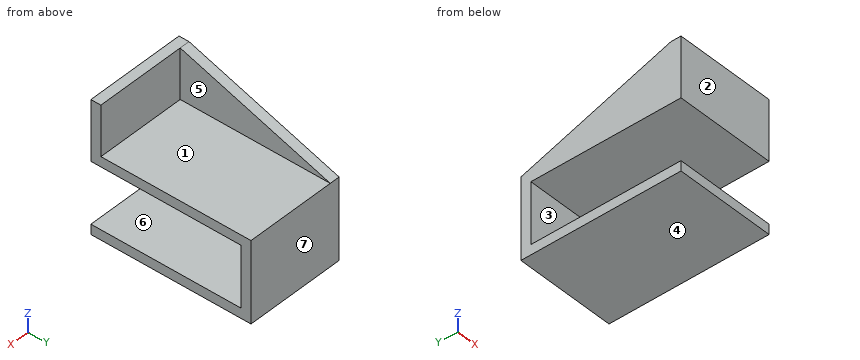
```python
from build123d import *

# Parameters (mm, degrees)
F0_W     = 25
F0_H     = 2.5
F1_DEPTH = 30.5
F2_W     = 50
F2_H     = 80
F3_DEPTH = 5
F4_W     = 50
F4_H     = 5
F5_DEPTH = 25
F7_DEPTH = 5
F8_W     = 50
F8_H     = 5
F9_DEPTH = 80


with BuildPart() as f1:
    # F0 (on Top) → F1 (new body)
    with BuildSketch(Plane.XY):
        with Locations((-12.5, 1.25)):
            Rectangle(F0_W, F0_H)
        with Locations((12.5, 1.25)):
            Rectangle(F0_W, F0_H)
        with Locations((-12.5, -1.25)):
            Rectangle(F0_W, F0_H)
        with Locations((12.5, -1.25)):
            Rectangle(F0_W, F0_H)
    extrude(amount=F1_DEPTH)

    # F2 (on face) → F3 (join)
    with BuildSketch(Plane.XY.offset(30.5)):
        with Locations((0, -37.5)):
            Rectangle(F2_W, F2_H)
    extrude(amount=F3_DEPTH)

    # F4 (on face) → F5 (join)
    with BuildSketch(Plane.XY.offset(35.5)):
        with Locations((0, -75)):
            Rectangle(F4_W, F4_H)
    extrude(amount=F5_DEPTH)

    # F6 (on face) → F7 (join)
    with BuildSketch(Plane(origin=(-25, 0, 0), x_dir=(0, -1, 0), z_dir=(-1, 0, 0))):
        Polygon((77.5, 30.5), (77.5, 60.5), (72.5, 60.5), (-2.5, 35.5), align=None)
    extrude(amount=-F7_DEPTH)

    # F8 (on face) → F9 (join, through all)
    with BuildSketch(Plane(origin=(0, 2.5, 0), x_dir=(-1, 0, 0), z_dir=(0, 1, 0))):
        with Locations((0, -2.5)):
            Rectangle(F8_W, F8_H)
    extrude(amount=-F9_DEPTH)


solid = f1.part
```
Geometry: final body of the model. Coordinates: model frame, mm. Face numbers are marked on the shaded views. A direction names the side the tool comes from. Round coordinates to 2 decimals unless told otherwise and drop trailing zeros. Loops run counter-clockwise (first coordinate to the right, second up) from the corner with the lowest first, then second, coordinate; pieces in that order, holes last.
Item 1: Section B-B, the plane y = -21.5. Output: boundary loops of the cut face in (x, z).
Checked values:
outline: (-25, -5) - (25, -5) - (25, 0) - (-25, 0) - close; (-25, 30.5) - (25, 30.5) - (25, 35.5) - (-20, 35.5) - (-20, 43.5) - (-25, 43.5) - close
Item 2: Line query: L1, parallel to Z at x = 21, y = -73; L2, parallel to Z at x = 7.5, y = -34; L3, parallel to Y at x = -7.5, z = 3. Output: solid intervals per line, ascending.
Checked values:
L1: z = -5 to 0, 30.5 to 60.5
L2: z = -5 to 0, 30.5 to 35.5
L3: y = -2.5 to 2.5
Item 3: Section A-A, the plane y = -8. Output: boundary loops of the cut face in (x, z).
Checked values:
outline: (-25, -5) - (25, -5) - (25, 0) - (-25, 0) - close; (-25, 30.5) - (25, 30.5) - (25, 35.5) - (-20, 35.5) - (-20, 39) - (-25, 39) - close
Item 4: Contact query for flat-ended pins moving along their axis: P1, Ø20, axis at x = 6.5, z = 48, coming from the +Y side; P2, Ø10, axis at x = -6, y = -43.5, coming from the +Z side; P3, Ø6, axis at y = -36.5, z = 49, coming from the +X side. Output: stop coordinate, or through.
Checked values:
P1: stops at y = -72.5
P2: stops at z = 35.5
P3: stops at x = -20
Item 5: Reachability of the marked faces 5, 6 and 7 from +Z, -Z, +X, -X, +Y, -Y: full face, straight path, thin tool, end or side. Return the list, or none.
Checked values:
face 5: +Z, +X, +Y
face 6: +X, -X, -Y
face 7: +Z, -Z, +X, -X, +Y
Item 6: Section C-C, the plane x = 7. Output: boundary loops of the cut face in (y, z), plus the area to 3 significant figures.
Checked values:
outline: (-77.5, -5) - (2.5, -5) - (2.5, 35.5) - (-72.5, 35.5) - (-72.5, 60.5) - (-77.5, 60.5) - (-77.5, 30.5) - (-2.5, 30.5) - (-2.5, 0) - (-77.5, 0) - close
area: 1,080 mm2
Item 7: Mould query, pull axis Z, two halves, no side actions, for the marked faces 1, 2, 3 and 4. Classes: released by +Z, released by -Z, zero draft, split by the parting line, or undercut.
Checked values:
face 1: released by +Z
face 2: zero draft
face 3: undercut
face 4: released by -Z
Item 8: Section D-D, the plane z = 54.5. Output: boundary loops of the cut face in (x, y), plus the area to 3 significant figures.
Checked values:
outline: (-25, -77.5) - (25, -77.5) - (25, -72.5) - (-20, -72.5) - (-20, -54.5) - (-25, -54.5) - close
area: 340 mm2
